The model under review builds one solid part; all positions refer to its coordinate system, in mm. A direction names the side the tool comes from. Give positions to 0.01 mm unless a question says otherwise; leave off trailing zeros. Order: outer loops, then holes, each group sorted by start corner. A loop starts at its lowest first (then second) coordinate and runs counter-clockwise, first axis right, second up. Notation, with made-up numbers: (50, 55.5) - (107, 55.5) arc R35 cw to (107, 93.5) - close; hole circle Ø7 at (-30, 63). An arc over 180 degrees is marked (long way). Use CSV: the item, a comma, the result in double quotes. Start each with the question number.
1. For pin 1 (3.5 mm diameter, centred on x = 113, y = 7, fed in from -Z); pin 2 (2.5 mm diameter, centred on y = 232, z = 5, fed in from +X); pin 3 (2.5 mm diameter, centred on y = 14.5, z = 2, fed in from -X); pin 4 (2.5 mm diameter, centred on x = -126, z = 2.5, fed in from -Y), all flat-tipped, find the tip position at first contact; note any pin that passes through.
2. Take a section at C-C, the plane y = 221.5. State the section outline as (x, z) points.
3. Take a section at B-B, the plane z = 4.75. Count the separate pieces of the cut face and the enclosed holes in it, then the cut area to 3 significant figures.
4. Machinability: for faces 5 (the flat face through (0, 13, 4)), 6 (the flat face through (-35, 152, 0)), 7 (the flat face through (-126, 250, 4)), which of the approach directions +Z, -Z, +X, -X, +Y, -Y give a long, thin tool a straight path to every point of the face, cutting with its end or side? Answer none if there is none.
5. Draft analysis for pull direction Y (two halves, no side actions). For faces 1 (the cylindrical face through (-101.745, 184.828, 3.944)), 2 (the flat face through (-30, 247, 4)), 3 (the flat face through (59, 0, 4)), 4 (the cylindrical face through (56.503, 8.154, 4.056)), state which applies: released by +Y, released by -Y, zero draft, split by the parting line, or undercut.
6. Take a section at D-D, the plane x = -23. State the section outline as (y, z) points, then the cut area to 3 significant figures.
7. Take a section at A-A, the plane x = -95. State the section outline as (y, z) points.
8. To check wall thickness, follow line 1 (X direction, y = 230, z = 3.25); line 2 (Y direction, x = -95, z = 6.5); line 3 (Y direction, x = 42.5, z = 5.5). State the ranges of each line that lie inside material, in increasing order. Write a range as [from, to].
```python
from build123d import *

# Parameters (mm, degrees)
F0_R     = 2
F0_R_2   = 8.5
F1_DEPTH = 8
F2_R     = 3.5
F3_DEPTH = 8
F4_R     = 5
F4_R_2   = 2
F5_DEPTH = 8
F6_R     = 10


with BuildPart() as f1:
    # F0 (on Top) → F1 (new body)
    with BuildSketch(Plane.XY):
        with BuildLine():
            Line((0, 30), (0, 0))
            Line((0, 0), (120, 0))
            Line((120, 0), (120, 51.421356))
            Line((120, 51.421356), (-30, 201.421356))
            Line((-30, 201.421356), (-30, 300))
            Line((-30, 300), (-130, 300))
            Line((-130, 300), (-130, 290.75))
            Line((-130, 290.75), (-126, 290.75))
            ThreePointArc((-126, 290.75), (-122.75, 287.5), (-126, 284.25))
            Line((-126, 284.25), (-130, 284.25))
            Line((-130, 284.25), (-130, 275))
            Line((-130, 275), (-122, 275))
            Line((-122, 275), (-122, 250))
            Line((-122, 250), (-130, 250))
            Line((-130, 250), (-130, 240.75))
            Line((-130, 240.75), (-126, 240.75))
            ThreePointArc((-126, 240.75), (-122.75, 237.5), (-126, 234.25))
            Line((-126, 234.25), (-130, 234.25))
            Line((-130, 234.25), (-130, 160))
            Line((-130, 160), (0, 30))
        make_face()
        with Locations((7, 7)):
            Circle(F0_R, mode=Mode.SUBTRACT)
        with Locations((41, 7)):
            Circle(F0_R, mode=Mode.SUBTRACT)
        with Locations((7, 43)):
            Circle(F0_R, mode=Mode.SUBTRACT)
        with Locations((41, 43)):
            Circle(F0_R, mode=Mode.SUBTRACT)
        with Locations((79, 7)):
            Circle(F0_R, mode=Mode.SUBTRACT)
        with Locations((113, 7)):
            Circle(F0_R, mode=Mode.SUBTRACT)
        with Locations((79, 43)):
            Circle(F0_R, mode=Mode.SUBTRACT)
        with Locations((113, 43)):
            Circle(F0_R, mode=Mode.SUBTRACT)
        with Locations((-115, 190)):
            Circle(F0_R, mode=Mode.SUBTRACT)
        with Locations((-95, 190)):
            Circle(F0_R_2, mode=Mode.SUBTRACT)
        with Locations((-75, 190)):
            Circle(F0_R, mode=Mode.SUBTRACT)
        with Locations((-115, 270)):
            Circle(F0_R, mode=Mode.SUBTRACT)
        with Locations((-95, 270)):
            Circle(F0_R_2, mode=Mode.SUBTRACT)
        with Locations((-75, 270)):
            Circle(F0_R, mode=Mode.SUBTRACT)
    extrude(amount=F1_DEPTH)

    # F2 (on face) → F3 (cut, through all)
    with BuildSketch(Plane.XY.offset(8)):
        with Locations((60, 8)):
            Circle(F2_R)
        with Locations((60, 40)):
            Circle(F2_R)
    extrude(amount=-F3_DEPTH, mode=Mode.SUBTRACT)

    # F4 (on face) → F5 (cut, through all)
    with BuildSketch(Plane(origin=(0, 0, 0), x_dir=(1, 0, 0), z_dir=(0, 0, -1))):
        with Locations((-95, -230)):
            Circle(F4_R)
        with Locations((-76.75, -230)):
            Circle(F4_R_2)
        with Locations((-113.25, -230)):
            Circle(F4_R_2)
    extrude(amount=-F5_DEPTH, mode=Mode.SUBTRACT)

    # F6
    f6_edges = [f1.edges().sort_by_distance(p)[0] for p in [
        (-130, 160, 4),
        (-30, 300, 4),
        (-30, 201.421356, 4),
        (120, 51.421356, 4),
        (0, 30, 4),
    ]]
    fillet(f6_edges, radius=F6_R)


solid = f1.part
```
Determined:
1,pin 1,"passes through"
1,pin 2,"stops at x = -30"
1,pin 3,"stops at x = 0"
1,pin 4,"stops at y = 154.75"
2,outline,"(-130, 0) - (-30, 0) - (-30, 8) - (-130, 8) - close"
3,separate pieces,"1"
3,enclosed holes,"19"
3,area,"35,500 mm²"
4,face 5,"+Z, -Z, -X, -Y"
4,face 6,"-Z, +X, -X, +Y, -Y"
4,face 7,"+Z, -Z, -X"
5,face 1,"undercut"
5,face 2,"zero draft"
5,face 3,"released by -Y"
5,face 4,"undercut"
6,outline,"(53, 0) - (194.42, 0) - (194.42, 8) - (53, 8) - close"
6,area,"1,130 mm²"
7,outline,"(125, 0) - (181.5, 0) - (181.5, 8) - (125, 8) - close; (198.5, 0) - (225, 0) - (225, 8) - (198.5, 8) - close; (235, 0) - (261.5, 0) - (261.5, 8) - (235, 8) - close; (278.5, 0) - (300, 0) - (300, 8) - (278.5, 8) - close"
8,line 1,"x = [-130, -115.25], [-111.25, -100], [-90, -78.75], [-74.75, -30]"
8,line 2,"y = [125, 181.5], [198.5, 225], [235, 261.5], [278.5, 300]"
8,line 3,"y = [0, 5.68], [8.32, 41.68], [44.32, 128.92]"
